Geometry: final body of the model. Coordinates: model frame, mm. A direction names the side the tool comes from. Give positions to 0.01 mm unless a question says otherwise; leave off trailing zeros. Write each loop counter-clockwise with the first axis right and the second up, starting at its lowest first coordinate (ties: lowest second). Pieces come first, ordered by that corner, then holes. Notation, with made-up numbers: M 75.5,8.5 L 89.5,8.5 A11 ccw 89.5,15.5 Z; hole C 32,-0.5 d9. An arc over 180 degrees is marked long. Answer as a JSON object with one key per item and string values.
from build123d import *

# Parameters (mm, degrees)
SKETCH_W     = 4
SKETCH_H     = 0.8
PAD_DEPTH    = 185
SKETCH002_W  = 8
SKETCH002_H  = 4
PAD001_DEPTH = 4


with BuildPart() as part:
    # Sketch → Pad (new body)
    with BuildSketch(Plane.XZ):
        Rectangle(SKETCH_W, SKETCH_H)
    extrude(amount=PAD_DEPTH)

    # Sketch002 (on Face4 of Pad) → Pad001 (join)
    with BuildSketch(Plane(origin=(0, 0, 0.4), x_dir=(-1, 0, 0), z_dir=(0, 0, 1))):
        with Locations((0, 183)):
            Rectangle(SKETCH002_W, SKETCH002_H)
        with Locations((0, 154.166667)):
            Rectangle(SKETCH002_W, SKETCH002_H)
        with Locations((0, 30.833333)):
            Rectangle(SKETCH002_W, SKETCH002_H)
        with Locations((0, 2)):
            Rectangle(SKETCH002_W, SKETCH002_H)
    extrude(amount=-PAD001_DEPTH)


solid = part.part
1) Cut plane A-A on z = -1.7. Return loops of the section in (x, y).
Geometry check:
{"outline": "M -4,-185 L 4,-185 L 4,-181 L -4,-181 Z; M -4,-156.17 L 4,-156.17 L 4,-152.17 L -4,-152.17 Z; M -4,-32.83 L 4,-32.83 L 4,-28.83 L -4,-28.83 Z; M -4,-4 L 4,-4 L 4,0 L -4,0 Z"}
2) Cut plane B-B on x = -0.75. Return loops of the section in (y, z), and give its area (3 significant figures).
Geometry check:
{"outline": "M -185,-3.6 L -181,-3.6 L -181,-0.4 L -156.17,-0.4 L -156.17,-3.6 L -152.17,-3.6 L -152.17,-0.4 L -32.83,-0.4 L -32.83,-3.6 L -28.83,-3.6 L -28.83,-0.4 L -4,-0.4 L -4,-3.6 L 0,-3.6 L 0,0.4 L -185,0.4 Z", "area": "199 mm2"}
3) Pull-direction query (Y, two-part tool) for faces 1 (the flat face through (0, -32.833, -2)), 2 (the flat face through (-4, -2, -2)), 3 (the flat face through (0, -185, -2)); classes: pulls with the +Y half, pulls with the -Y half, needs draft (parallel to the pull), parting line crosses it, or undercut.
Geometry check:
{"face 1": "undercut", "face 2": "needs draft", "face 3": "pulls with the -Y half"}
4) Cut plane C-C on y = -172. Return loops of the section in (x, z), and give its area (3 significant figures).
Geometry check:
{"outline": "M -2,-0.4 L 2,-0.4 L 2,0.4 L -2,0.4 Z", "area": "3.20 mm2"}
5) Set-up query: faces 4 (the flat face through (0, -168, -0.4)), 5 (the flat face through (0, -94, 0.4)). Return all of +Z, -Z, +X, -X, +Y, -Y with unobstructed straight access to the full face (end or side cutting, diameter ignored); none if empty.
Geometry check:
{"face 4": "-Z, +X, -X", "face 5": "+Z, +X, -X, +Y, -Y"}
6) Contact query for flat-ended pins moving along their axis: P1, Ø0.9, axis at y = -18.5, z = 0, coming from the +X side; P2, Ø1.2, axis at x = -0.5, y = -19.5, coming from the -Z side; P3, Ø0.6, axis at y = -19.5, z = 0, coming from the -X side; P4, Ø2, axis at y = -148, z = -1.5, coming from the +X side. Output: stop coordinate, or through.
Geometry check:
{"P1": "stops at x = 2", "P2": "stops at z = -0.4", "P3": "stops at x = -2", "P4": "passes through"}
7) Line query: line 1 (Y direction, x = -1, z = -2.8); line 2 (Z direction, x = 1.75, y = -163); line 3 (X direction, y = -81.5, z = 0.2). Output: solid intervals per line, ascending. Write a range as from..to.
Geometry check:
{"line 1": "y = -185..-181, -156.17..-152.17, -32.83..-28.83, -4..0", "line 2": "z = -0.4..0.4", "line 3": "x = -2..2"}
